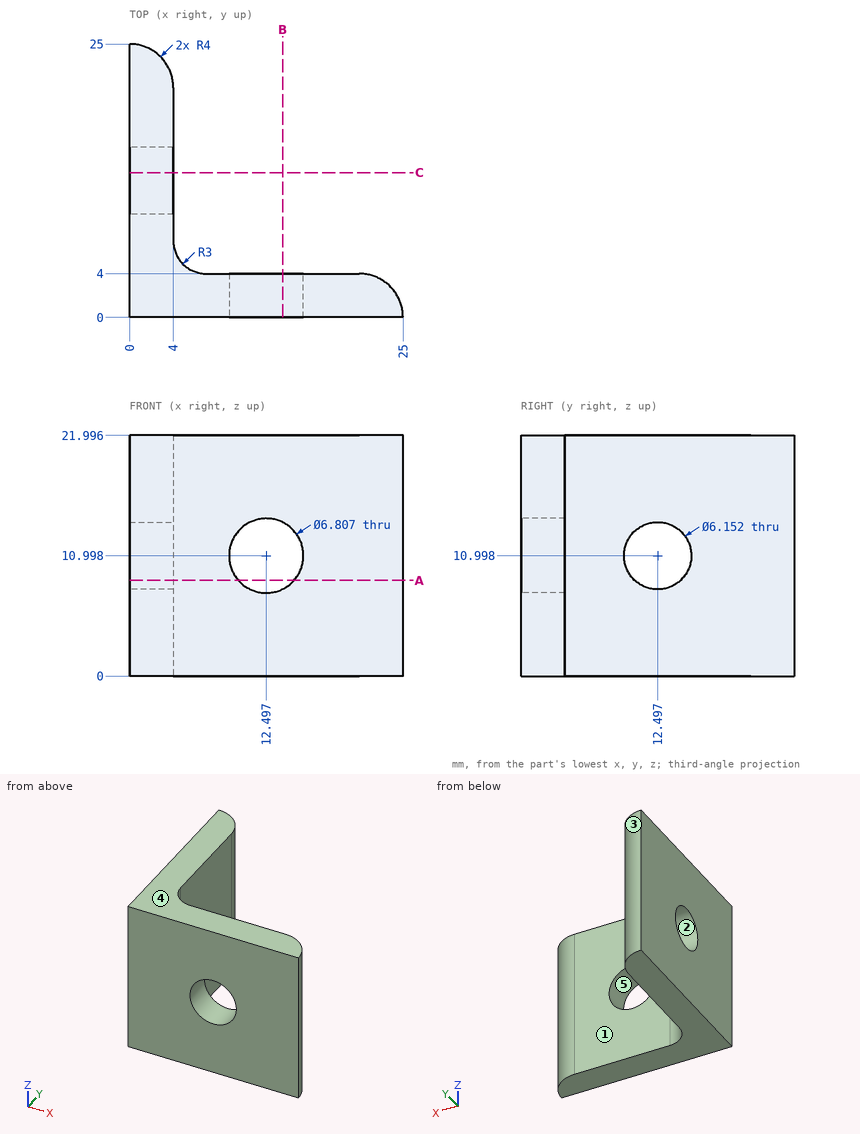
Here's the drawing with two shaded views (mm, measured from the low corner). I have some questions. A direction names the side the tool comes from. Coordinates: 2 decimals unless noted, no trailing zeros. Order: outer loops, then holes, each group sorted by start corner. A loop starts at its lowest first (then second) coordinate and runs counter-clockwise, first axis right, second up. Notation, with made-up numbers: (-34, 36) -> (24, 36) arc R20 ccw to (24, 62) -> close; hole circle Ø11 at (36.25, 0). An arc over 180 degrees is marked (long way). One line per question, with ' | ' between items.
Q1. Imagine slicing it at B-B on x = 14. Please give me the cut outline in (y, z) (1 decimal).
Return value:
outline: (0, 0) -> (4, 0) -> (4, 7.9) -> (0, 7.9) -> close; (0, 14.1) -> (4, 14.1) -> (4, 22) -> (0, 22) -> close
Q2. If I drill on L1, parallel to Y at x = 9.75, z = 2.75; L2, parallel to X at y = 22.5, z = 11, over which ranges is the centre line in solid material (lowest first)?
Return value:
L1: 0 to 4 | L2: 0 to 3.71
Q3. On a 3-axis mill with a long thin cutter (end or side, diameter ignored), from which of +Z, -Z, +X, -X, +Y, -Y can I reach the whole of each face in a straight line? I mean the marked faces 1 and 2. Say none if no direction works.
Return value:
face 1: +Z, -Z, +X, +Y | face 2: +X, -X
Q4. I'm going to push flat-ended pins straight in: P1, Ø8, axis at y = 12.5, z = 11, coming from the -X side; P2, Ø4, axis at x = 12, z = 8, coming from the +Y side; P3, Ø4, axis at y = 11, z = 16.5, coming from the +X side. Where does each tip first touch, or does it pass through?
Return value:
P1: x = 0 | P2: y = 4 | P3: x = 4
Q5. Thinking about a two-plate mould opening in Z: for the marked faces 3, 4 and 5, which applies, pulls with the +Z half, pulls with the -Z half, needs draft (parallel to the pull), parting line crosses it, or undercut?
Return value:
face 3: needs draft | face 4: pulls with the +Z half | face 5: undercut
Q6. Imagine slicing it at A-A on z = 8.75. State how many separate pieces and enclosed holes the cut face has, and give its area (3 significant figures).
Return value:
separate pieces: 3 | enclosed holes: 0 | area: 142 mm²
Q7. Imagine slicing it at C-C on y = 13.25. Please give me the cut outline in (x, z).
Return value:
outline: (0, 0) -> (4, 0) -> (4, 8.02) -> (0, 8.02) -> close; (0, 13.98) -> (4, 13.98) -> (4, 22) -> (0, 22) -> close
